from build123d import *

# Parameters (mm, degrees)
SKETCH2_R                              = 14
BOSS_EXTRUDE1_DEPTH                    = 3
SKETCH3_R                              = 6
BOSS_EXTRUDE2_DEPTH                    = 26.5
BOSS_EXTRUDE3_DEPTH                    = 1
M36_CLEARANCE_HOLE1_D                  = 39
M36_CLEARANCE_HOLE1_DEPTH              = 4.45
F_1_5_1_5_DIAMETER_HOLE1_D             = 1.5
F_1_5_1_5_DIAMETER_HOLE1_DEPTH         = 2
F_1_5_1_5_DIAMETER_HOLE1_TIP           = 0.450645464
F_3_3_3_3_DIAMETER_HOLE1_D             = 3.3
F_3_3_3_3_DIAMETER_HOLE1_DEPTH         = 6
F_3_3_3_3_DIAMETER_HOLE1_TIP           = 0.991420021
F_1_25_1_25_DIAMETER_HOLE1_D           = 1.25
F_1_25_1_25_DIAMETER_HOLE1_DEPTH       = 1.939156082
F_1_25_1_25_DIAMETER_HOLE1_CSINK_D     = 2.65
F_1_25_1_25_DIAMETER_HOLE1_CSINK_ANGLE = 60
F_1_25_1_25_DIAMETER_HOLE1_TIP         = 0.360843918
CHAMFER1_SIZE                          = 0.288675135
CHAMFER1_SIZE2                         = 0.5


with BuildPart() as part:
    # Sketch1 → Revolve1 (revolve)
    with BuildSketch(Plane.XY, mode=Mode.PRIVATE) as revolve1_sk:
        with BuildLine():
            Line((0, 21), (0, 0))
            Line((0, 0), (41, 0))
            Line((41, 0), (41, 21))
            Line((41, 21), (9.25, 21))
            ThreePointArc((9.25, 21), (9.2, 20.98660254), (9.15, 21))
            Line((9.15, 21), (0, 21))
        make_face()
    revolve(revolve1_sk.sketch.rotate(Axis((0, 0, 0), (1, 0, 0)), 270), axis=Axis((0, 0, 0), (1, 0, 0)))

    # Sketch2 → Boss-Extrude1 (add)
    with BuildSketch(Plane.ZY):
        Circle(SKETCH2_R)
    extrude(amount=BOSS_EXTRUDE1_DEPTH)

    # Sketch3 → Boss-Extrude2 (add)
    with BuildSketch(Plane.ZY.offset(3)):
        Circle(SKETCH3_R)
    extrude(amount=BOSS_EXTRUDE2_DEPTH)

    # Sketch4 → Boss-Extrude3 (add)
    with BuildSketch(Plane.ZY.offset(3)):
        with BuildLine():
            Line((0.293916284, -7.616838781), (0.293916284, -5.992796778))
            ThreePointArc((0.293916284, -5.992796778), (0, 6), (-0.293916284, -5.992796778))
            Line((-0.293916284, -5.992796778), (-0.293916284, -7.616838781))
            ThreePointArc((-0.293916284, -7.616838781), (-1.755912185, -7.072113956), (-2.882513969, -5.992796778))
            ThreePointArc((-2.882513969, -5.992796778), (0, 6.65), (2.882513969, -5.992796778))
            ThreePointArc((2.882513969, -5.992796778), (1.821852016, -7.17721696), (0.293916284, -7.616838781))
        make_face()
    extrude(amount=BOSS_EXTRUDE3_DEPTH)

    # M36 Clearance Hole1
    with Locations(Plane(origin=(41, 0, 0), x_dir=(0, 0, -1), z_dir=(1, 0, 0))):
        with Locations((0, 0)):
            Hole(M36_CLEARANCE_HOLE1_D / 2, depth=M36_CLEARANCE_HOLE1_DEPTH)

    # Ø1.5 (1.5) Diameter Hole1
    with Locations(Plane.ZY):
        with Locations((-7.462326931, 18.015650884)):
            Hole(F_1_5_1_5_DIAMETER_HOLE1_D / 2, depth=F_1_5_1_5_DIAMETER_HOLE1_DEPTH)
            with Locations((0, 0, -(F_1_5_1_5_DIAMETER_HOLE1_DEPTH + F_1_5_1_5_DIAMETER_HOLE1_TIP / 2))):  # 118° drill point
                Cone(0, F_1_5_1_5_DIAMETER_HOLE1_D / 2, F_1_5_1_5_DIAMETER_HOLE1_TIP, mode=Mode.SUBTRACT)

    # Ø3.3 (3.3) Diameter Hole1
    with Locations(Plane.ZY):
        with Locations((3.0543e-05, 17.5), (17.5, -3.0543e-05), (-3.0543e-05, -17.5), (-17.5, 3.0543e-05)):
            Hole(F_3_3_3_3_DIAMETER_HOLE1_D / 2, depth=F_3_3_3_3_DIAMETER_HOLE1_DEPTH)
            with Locations((0, 0, -(F_3_3_3_3_DIAMETER_HOLE1_DEPTH + F_3_3_3_3_DIAMETER_HOLE1_TIP / 2))):  # 118° drill point
                Cone(0, F_3_3_3_3_DIAMETER_HOLE1_D / 2, F_3_3_3_3_DIAMETER_HOLE1_TIP, mode=Mode.SUBTRACT)

    # Ø1.25 (1.25) Diameter Hole1
    with Locations(Plane.ZY.offset(29.5)):
        with Locations((0, 0)):
            CounterSinkHole(F_1_25_1_25_DIAMETER_HOLE1_D / 2, F_1_25_1_25_DIAMETER_HOLE1_CSINK_D / 2, depth=F_1_25_1_25_DIAMETER_HOLE1_DEPTH, counter_sink_angle=F_1_25_1_25_DIAMETER_HOLE1_CSINK_ANGLE)
            with Locations((0, 0, -(F_1_25_1_25_DIAMETER_HOLE1_DEPTH + F_1_25_1_25_DIAMETER_HOLE1_TIP / 2))):  # 120° drill point
                Cone(0, F_1_25_1_25_DIAMETER_HOLE1_D / 2, F_1_25_1_25_DIAMETER_HOLE1_TIP, mode=Mode.SUBTRACT)

    # Chamfer1
    chamfer1_edges = [part.edges().sort_by_distance(p)[0] for p in [
        (-29.5, 0, -6),
    ]]
    chamfer1_side = [part.faces().sort_by_distance(p)[0] for p in [
        (-29.5, 0, -5.830294373),
    ]]
    chamfer(chamfer1_edges, length=CHAMFER1_SIZE, length2=CHAMFER1_SIZE2, reference=chamfer1_side[0])


solid = part.part
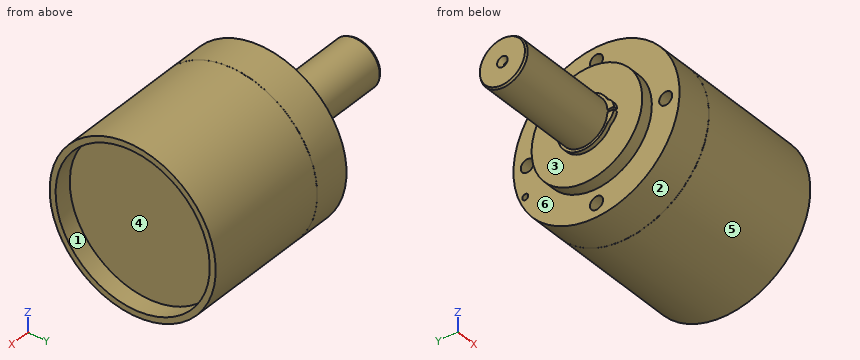
Verification items for the finished model (mm, model axes). Face numbers are marked on the shaded views. A direction names the side the tool comes from. Give positions to 0.01 mm unless a question says otherwise; leave off trailing zeros. Write each loop counter-clockwise with the first axis right and the second up, starting at its lowest first coordinate (ties: lowest second). Pieces come first, ordered by that corner, then holes.
(1) Mould release check, pull along Y, two halves, no side actions. Record for the marked faces 1, 2 and 3: +Y half, -Y half, draft (parallel to the pull), parting line (faces both ways), or undercut.
(2) Material ranges on line 1 (Y direction, x = -28, z = 0) (3 decimals); line 2 (Z direction, x = -27, y = 0); line 3 (X direction, y = -12.5, z = 11.5), recorded low to high.
(3) Cross-section at A-A (x = 3.5). Enter the section's corners in (y, z), plus the area to 3 significant figures.
(4) Cross-section at B-B (x = 20.5). Enter the section's corners in (y, z).
(5) Access from +Z, -Z, +X, -X, +Y, -Y to the whole of each face (thin tool, end or side, straight path). Record for the marked faces 4, 5 and 6.
(6) Gauge pin test, flat ends, axial feed: pin 1 (2.5 mm diameter, centred on y = -17.5, z = 0, fed in from +X); pin 2 (12 mm diameter, centred on x = 12.5, y = 12.5, fed in from +Z); pin 3 (2 mm diameter, centred on y = 18.02, z = -7.46, fed in from -X). Record the tip position at first contact, or that the pin passes through.
Worked out:
1. face 1: undercut
1. face 2: parting line
1. face 3: draft
2. line 1: y = -6 to -0.625, 0.625 to 6
2. line 2: z = -6 to 6
2. line 3: x = 0 to 36.55
3. outline: circle Ø42 at (0, 0); hole circle Ø3.3 at (-17.5, 0); hole circle Ø3.3 at (0, -17.5); hole circle Ø3.3 at (0, 17.5); hole circle Ø3.3 at (17.5, 0)
3. area: 1,350 mm2
4. outline: circle Ø42 at (0, 0)
5. face 4: +X
5. face 5: +X, -X
5. face 6: -X
6. pin 1: stops at x = 36.55
6. pin 2: stops at z = 19.97
6. pin 3: stops at x = 0
